The model under review builds one solid part; all positions refer to its coordinate system, in mm. A direction names the side the tool comes from. Round coordinates to 2 decimals unless told otherwise and drop trailing zeros. Order: outer loops, then holes, each group sorted by start corner. A loop starts at its lowest first (then second) coordinate and runs counter-clockwise, first axis right, second up. Notation, with made-up numbers: M -17,74.5 L 35,74.5 A21 cw 35,78.5 Z; hole C -16.5,-0.5 d11. An arc over 180 degrees is marked long. Answer as a JSON object with one key per item and string values. Group by question number.
1) For faces 1 (the flat face through (975, -1, -7.62)), 2 (the flat face through (-976, -1, -7.62)), 3 (the flat face through (-13, -1, -12.7)), list the 3-axis set-ups (+Z, -Z, +X, -X, +Y, -Y) from which the entire face can be reached by the end or side of a thin tool; tool diameter is ignored.
2) Consider section A-A, the plane x = -187. Write out the cut boundary in (y, z), then the cut area to 3 significant figures.
3) Consider section B-B, the plane y = 8. Write out the cut boundary in (x, z), then the cut area to 3 significant figures.
4) Insertion check: pin 1 Ø3 at (x, z) = (481.5, -8) entering from -Y; pin 2 Ø4 at (x, z) = (494, 3) entering from +Y; pin 3 Ø2.5 at (y, z) = (20.5, -11) entering from -X. Each pin has a flat end and moves straight along its axis. Give the tip position at first contact, or say it passes through.
5) To check wall thickness, follow line 1 (Y direction, x = 29.5, z = 3.75); line 2 (Y direction, x = -270, z = 6.5); line 3 (X direction, y = 8, z = -9.25). State the ranges of each line that lie inside material, in increasing order.
```python
from build123d import *

# Parameters (mm, degrees)
BOSS_EXTRUDE2_DEPTH     = 1021.08
FILLET1_R               = 2.54
CUT_EXTRUDE1_DEPTH      = 1023.421780089
CUT_EXTRUDE1_DEPTH_BACK = 1023.421780089
SKETCH2_W               = 91.44
SKETCH2_H               = 5.08


with BuildPart() as part:
    # Sketch1 → Boss-Extrude2 (new, symmetric)
    with BuildSketch(Plane(origin=(0, 0, 0), x_dir=(0, 0, -1), z_dir=(1, 0, 0))):
        with BuildLine():
            ThreePointArc((-12.7, -47.397045256), (-6.574003886, -49.93451595), (-2.91e-07, -50.8))
            ThreePointArc((-2.91e-07, -50.8), (6.574003605, -49.934516025), (12.7, -47.397045256))
            Line((12.7, -47.397045256), (12.7, 47.397045256))
            ThreePointArc((12.7, 47.397045256), (6.574003746, 49.934515988), (0, 50.8))
            ThreePointArc((0, 50.8), (-6.574003746, 49.934515988), (-12.7, 47.397045256))
            Line((-12.7, 47.397045256), (-12.7, -47.397045256))
        make_face()
    extrude(amount=BOSS_EXTRUDE2_DEPTH, both=True)

    # Fillet1
    fillet1_edges = [part.edges().sort_by_distance(p)[0] for p in [
        (-510.54, 47.397045256, 12.7),
        (510.54, 47.397045256, -12.7),
        (-510.54, -47.397045256, -12.7),
        (0, -47.397045256, 12.7),
    ]]
    fillet(fillet1_edges, radius=FILLET1_R)

    # Sketch2 → Cut-Extrude1 (cut, two sides: drawn at the far end of the back side and taken through both)
    with BuildSketch(Plane(origin=(0, 0, 0), x_dir=(1, 0, 0), z_dir=(0, 1, 0)).offset(-CUT_EXTRUDE1_DEPTH_BACK)):
        with Locations((975.36, 10.16)):
            Rectangle(SKETCH2_W, SKETCH2_H)
        with Locations((-975.36, 10.16)):
            Rectangle(SKETCH2_W, SKETCH2_H)
    extrude(amount=CUT_EXTRUDE1_DEPTH + CUT_EXTRUDE1_DEPTH_BACK, mode=Mode.SUBTRACT)


solid = part.part
```
Results list:
{
 "1": {"face 1": "-Z, +X, +Y, -Y", "face 2": "-Z, -X, +Y, -Y", "face 3": "-Z, +X, -X, +Y, -Y"},
 "2": {"outline": "M -48.15,-11.29 A2.54 ccw -45.88,-12.7 L 45.88,-12.7 A2.54 ccw 48.15,-11.29 A25.4 ccw 48.15,11.29 A2.54 ccw 45.88,12.7 L -45.88,12.7 A2.54 ccw -48.15,11.29 A25.4 ccw Z", "area": "2,520 mm^2"},
 "3": {"outline": "M -1021.08,-7.62 L -929.64,-7.62 L -929.64,-12.7 L 929.64,-12.7 L 929.64,-7.62 L 1021.08,-7.62 L 1021.08,12.7 L -1021.08,12.7 Z", "area": "50,900 mm^2"},
 "4": {"pin 1": "y = -49.95", "pin 2": "y = 50.78", "pin 3": "x = -929.64"},
 "5": {"line 1": "-50.52 to 50.52", "line 2": "-49.95 to 49.95", "line 3": "-929.64 to 929.64"}
}
